from build123d import *

# Parameters (mm, degrees)
F4_R     = 5
F5_DEPTH = 2.5


with BuildPart() as f2:
    # F2: sweep along a path in F0
    with BuildLine(Plane.XZ) as f2_path:
        Line((0, 60), (-90, 60))
        ThreePointArc((-90, 60), (-97.071068, 57.071068), (-100, 50))
        Line((-100, 50), (-100, 0))
    # F1 (on Right) → F2 (sweep)
    with BuildSketch(Plane.YZ):
        with BuildLine():
            Line((-10, 100), (-10, 95))
            Line((-10, 95), (-5.5, 95))
            ThreePointArc((-5.5, 95), (-3.37868, 94.12132), (-2.5, 92))
            Line((-2.5, 92), (-2.5, 68))
            ThreePointArc((-2.5, 68), (-3.37868, 65.87868), (-5.5, 65))
            Line((-5.5, 65), (-10, 65))
            Line((-10, 65), (-10, 60))
            Line((-10, 60), (0, 60))
            Line((0, 60), (10, 60))
            Line((10, 60), (10, 65))
            Line((10, 65), (5.5, 65))
            ThreePointArc((5.5, 65), (3.37868, 65.87868), (2.5, 68))
            Line((2.5, 68), (2.5, 92))
            ThreePointArc((2.5, 92), (3.37868, 94.12132), (5.5, 95))
            Line((5.5, 95), (10, 95))
            Line((10, 95), (10, 100))
            Line((10, 100), (-10, 100))
        make_face()
    sweep(path=f2_path.line)

    # F3: F2 across plane


with BuildPart() as f2_1:
    add(f2.part)
    add(f2.part.mirror(Plane.XY))

    # F4 (on Front) → F5 (join, symmetric)
    with BuildSketch(Plane.XZ):
        with BuildLine():
            Line((-35.548045, 142.580075), (-70, 100))
            Line((-70, 100), (0, 100))
            Line((0, 100), (0, 130))
            ThreePointArc((0, 130), (-13.327703, 148.854189), (-35.548045, 142.580075))
        make_face()
        with Locations((-20, 130)):
            Circle(F4_R, mode=Mode.SUBTRACT)
        with BuildLine():
            Line((0, -100), (-70, -100))
            Line((-70, -100), (-35.548045, -142.580075))
            ThreePointArc((-35.548045, -142.580075), (-13.327703, -148.854189), (0, -130))
            Line((0, -130), (0, -100))
        make_face()
        with Locations((-20, -130)):
            Circle(F4_R, mode=Mode.SUBTRACT)
    extrude(amount=F5_DEPTH, both=True)


solid = f2_1.part
The listing builds one solid part. Answer for the finished solid, in the listing's coordinates (mm). A direction names the side the tool comes from. Coordinates: 2 decimals unless noted, no trailing zeros. Order: outer loops, then holes, each group sorted by start corner. A loop starts at its lowest first (then second) coordinate and runs counter-clockwise, first axis right, second up. Notation, with made-up numbers: (4.5, 0.25) -> (54.5, 0.25) arc R14 ccw to (54.5, 21.25) -> close; hole circle Ø3 at (-19.75, -1). An arc over 180 degrees is marked (long way). Answer in a Markdown table with one row per item. Add a question column.
Item 1: Which of the six approach directions +Z, -Z, +X, -X, +Y, -Y give full straight-line access (tool end or side, diameter ignored) to faces 5 (the face through (-121.468, -7.719, -82.168)), 6 (the face through (-100, 0, 1)), 7 (the face through (-28, 2.5, -119))?
Item 2: Find section B-B (x = -20). State how many separate pieces and enclosed holes the cut face has, then the cut area to 3 significant figures.
Item 3: Each of these flat-tipped pins is pushed along its axis until it touches: P1, Ø2, axis at x = -64.5, y = 7, coming from the -Z side; P2, Ø25, axis at x = -18.5, z = 129, coming from the -Y side; P3, Ø1.5, axis at x = -115, y = -6.5, coming from the -Z side. Where does it stop, or does it pass through?
Item 4: Determine the mould class of faces 1 (the face through (-124.964, -0.14, 85.742)), 2 (the face through (-121.468, 7.782, 82.168)), 3 (the face through (-13.654, -0.035, -148.966)), 4 (the face through (-46, 0, 60)) for opening direction Z: +Z half, -Z half, draft (parallel to the pull), parting line (faces both ways), or undercut.
Item 5: Find the intervals of material crossed by L1, parallel to Z at x = -20, y = -0.2; L2, parallel to Z at x = -49.5, y = -5; L3, parallel to X at y = 8.5, z = -34, in increasing order. Write a range as from..to.
Item 6: Find section C-C (z = -110.5). Write down the section's boundary in (x, y).
Result set:
| question | item | result |
|---|---|---|
| 1 | face 5 | -Y |
| 1 | face 6 | +X, +Y, -Y |
| 1 | face 7 | -Z, +X, -X, +Y |
| 2 | separate pieces | 4 |
| 2 | enclosed holes | 0 |
| 2 | area | 1,120 mm² |
| 3 | P1 | stops at z = -100 |
| 3 | P2 | stops at y = -2.5 |
| 3 | P3 | stops at z = -93.73 |
| 4 | face 1 | +Z half |
| 4 | face 2 | undercut |
| 4 | face 3 | -Z half |
| 4 | face 4 | undercut |
| 5 | L1 | z = -150..-135, -125..-60, 60..125, 135..150 |
| 5 | L2 | z = -100..-94.96, -65.04..-60, 60..65.04, 94.96..100 |
| 5 | L3 | x = -140..-135, -105..-100 |
| 6 | outline | (-61.5, -2.5) -> (0, -2.5) -> (0, 2.5) -> (-61.5, 2.5) -> close |
